Design review of the part built by this model. Coordinates are the model's own, in mm. Coordinates: 2 decimals unless noted, no trailing zeros. Write each loop counter-clockwise with the first axis right and the second up, starting at its lowest first coordinate (ties: lowest second). Pieces come first, ordered by that corner, then holes.
Q1. Take a section at A-A, the plane z = -18.5. Write out the cut boundary in (x, y).
Q2. The part is to be moulded in two halves that separate along Z. For faces 1 (the flat face through (-0.333, -9.448, 27.711)), 2 (the flat face through (9.09, 5.25, 13)), say which applies: released by +Z, released by -Z, zero draft, split by the parting line, or undercut.
Q3. For L1, parallel to X at y = 12.5, z = 22; L2, parallel to X at y = 3, z = 54.5; L3, parallel to Y at x = 16.5, z = 25, list the stretches that pass through material, from the lowest coordinate up.
Q4. For pin 1 Ø12 at (x, y) = (13, -9) entering from +Z; pin 2 Ø2 at (x, y) = (-9.5, -12.5) entering from +Z; pin 3 Ø1 at (x, z) = (14.5, -15) entering from +Y, all flat-tipped, find the tip position at first contact; note any pin that passes through.
from build123d import *

# Parameters (mm, degrees)
F1_ANGLE_BACK = 260
F1_ANGLE      = 290
F4_DEPTH      = 80


with BuildPart() as f1:
    # F0 (on Front) → F1 (revolve)
    with BuildSketch(Plane.XZ, mode=Mode.PRIVATE) as f1_sk:
        with BuildLine():
            Line((0, 70.9821507335), (0, 25))
            ThreePointArc((0, 25), (17.6776695297, 17.6776695297), (25, 0))
            add(Edge.make_bspline(
                [(25, 0), (25.7729905135, 10.449231781), (27.4753426857, 33.4615095623), (9.7026241041, 57.7321366539), (0, 70.9821507335)],
                knots=[0, 0, 0, 0, 0.4540720341, 1, 1, 1, 1], degree=3))
        make_face()
        with BuildLine():
            Line((0, 25), (0, -25))
            ThreePointArc((0, -25), (17.6776695297, -17.6776695297), (25, 0))
            ThreePointArc((25, 0), (17.6776695297, 17.6776695297), (0, 25))
        make_face()
    revolve(f1_sk.sketch.rotate(Axis((0, 0, 22.9910753667), (0, 0, 1)), -F1_ANGLE_BACK), axis=Axis((0, 0, 22.9910753667), (0, 0, 1)), revolution_arc=F1_ANGLE)

    # F3 (on offset) → F4 (cut)
    with BuildSketch(Plane.YZ.offset(-50)):
        Polygon((-15.8244016312, 19.0178565681), (-8.8184551604, 19.0178565681), (-6.6534986392, 25.680907612), (-12.3214283958, 29.7988996259), (-17.9893581524, 25.680907612), align=None)
    extrude(amount=F4_DEPTH, mode=Mode.SUBTRACT)


solid = f1.part
Responses:
1. outline: (-2.92, 16.56) arc R16.82 ccw (long way) to (14.56, 8.41) - (0, 0) - close
2. face 1: undercut
2. face 2: zero draft
3. L1: x = -21.94 to -2.2, 21.65 to 21.94
3. L2: x = -11.28 to -0.53, 5.2 to 11.28
3. L3: y = -18.56 to -17.77, -6.87 to 9.53
4. pin 1: stops at z = 57.27
4. pin 2: stops at z = 49.75
4. pin 3: stops at y = 8.66
